For this review, take the finished solid that the model builds, in its own axes (mm). A direction names the side the tool comes from. Give positions to 0.01 mm unless a question says otherwise; leave off trailing zeros. Loops run counter-clockwise (first coordinate to the right, second up) from the corner with the lowest first, then second, coordinate; pieces in that order, holes last. Notation, with made-up numbers: (48, 55) -> (95, 55) arc R30 cw to (95, 93) -> close; hole circle Ø3 at (86, -6). An arc over 180 degrees is marked (long way). Write each question's results on one line, items separated by ' | '. Start each with the question number.
```python
from build123d import *

# Parameters (mm, degrees)
SKETCH1_W                = 47
SKETCH1_H                = 40
BOSS_EXTRUDE1_DEPTH      = 4.5
FILLET1_R                = 1
SKETCH2_W                = 3
SKETCH2_H                = 4.5
BOSS_EXTRUDE2_DEPTH      = 3
BOSS_EXTRUDE2_DEPTH_BACK = 3


with BuildPart() as part:
    # Sketch1 → Boss-Extrude1 (new body)
    with BuildSketch(Plane(origin=(0, 0, 0), x_dir=(1, 0, 0), z_dir=(0, 1, 0))):
        Rectangle(SKETCH1_W, SKETCH1_H)
    extrude(amount=BOSS_EXTRUDE1_DEPTH)

    # Fillet1
    fillet1_edges = [part.edges().sort_by_distance(p)[0] for p in [
        (0, 4.5, -20),
        (0, 0, -20),
        (0, 0, 20),
        (0, 4.5, 20),
    ]]
    fillet(fillet1_edges, radius=FILLET1_R)

    # Sketch2 → Boss-Extrude2 (add, two sides)
    with BuildSketch(Plane.XY.offset(20)) as boss_extrude2_sk:
        with Locations((-22, 2.25)):
            Rectangle(SKETCH2_W, SKETCH2_H)
    extrude(amount=BOSS_EXTRUDE2_DEPTH)
    extrude(boss_extrude2_sk.sketch, amount=-BOSS_EXTRUDE2_DEPTH_BACK)


solid = part.part
```
1. For pin 1 Ø2 at (x, y) = (4, 2) entering from +Z, flat-tipped, find the tip position at first contact; note if it passes through.
2. Machinability: for faces 1 (the flat face through (1, 2, 20)), 2 (the cylindrical face through (1.808, 0.301, 19.715)), 3 (the cylindrical face through (1.808, 4.199, 19.715)), which of the approach directions +Z, -Z, +X, -X, +Y, -Y give a long, thin tool a straight path to every point of the face, cutting with its end or side? Answer none if there is none.
3. We need section B-B (y = 2.1). Write out the cut boundary in (x, z), plus the area to 3 significant figures.
4. We need section A-A (x = -1.5). Write out the cut boundary in (y, z).
5. Wall thickness on L1, parallel to Z at x = -20, y = 1.7; L2, parallel to Z at x = -4, y = 0.5; L3, parallel to Y at x = 5.5, z = 19.5: over which ranges is each line inside the solid? List them lowest first.
Response:
1) pin 1: stops at z = 20
2) face 1: +Z, +X, +Y, -Y | face 2: +Z, +X, -Y | face 3: +Z, +X, +Y
3) outline: (-23.5, -20) -> (23.5, -20) -> (23.5, 20) -> (-20.5, 20) -> (-20.5, 23) -> (-23.5, 23) -> close | area: 1,890 mm2
4) outline: (0, -19) arc R1 ccw to (1, -20) -> (3.5, -20) arc R1 ccw to (4.5, -19) -> (4.5, 19) arc R1 ccw to (3.5, 20) -> (1, 20) arc R1 ccw to (0, 19) -> close
5) L1: z = -20 to 20 | L2: z = -19.87 to 19.87 | L3: y = 0.13 to 4.37
